For this review, use the dimensioned drawing (mm, ordinates from the lowest corner) and the shaded views. A direction names the side the tool comes from. Coordinates: 2 decimals unless noted, no trailing zeros. Order: outer loops, then holes, each group sorted by start corner. A loop starts at its lowest first (then second) coordinate and runs counter-clockwise, first axis right, second up. Notation, with made-up numbers: M 48,84 L 86,84 A27 ccw 86,106 Z; hole C 76,48.25 d9. An arc over 180 degrees is marked long. Answer in a Markdown table with one row per item.
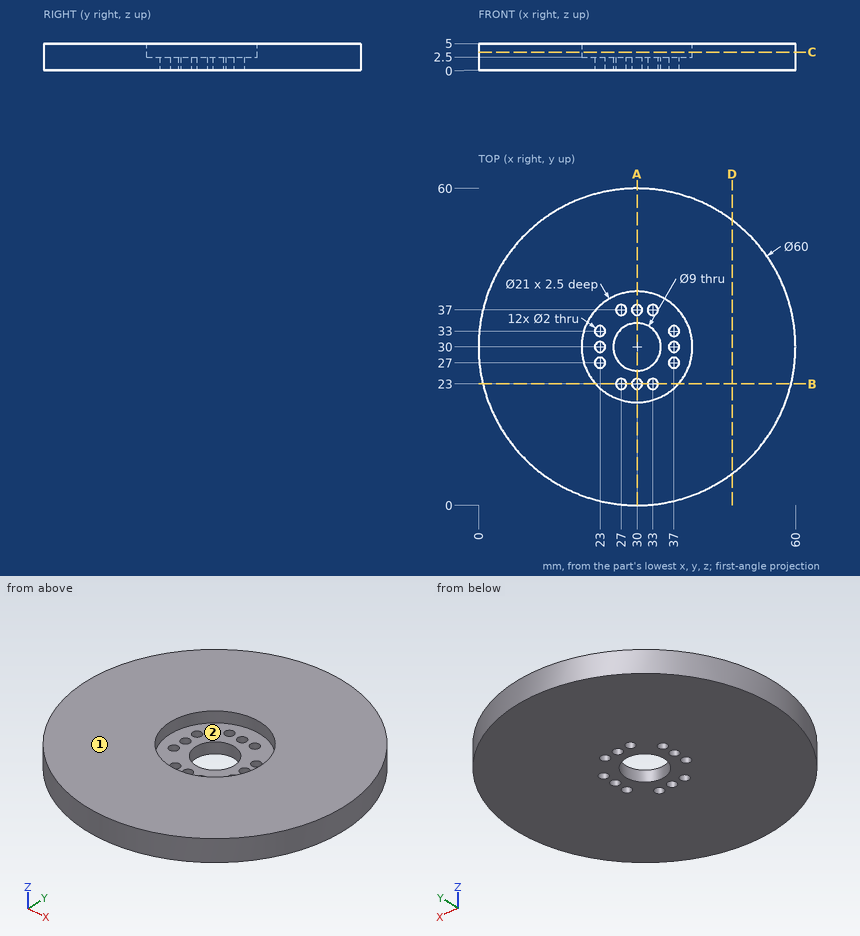
(1) Add section D-D, the plane x = 48. Give the boundary of the cut face in (y, z).
Return value:
| item | result |
|---|---|
| outline | M 6,0 L 54,0 L 54,5 L 6,5 Z |
(2) Insertion check: pin 1 Ø5.5 at (x, y) = (30, 30) entering from +Z; pin 2 Ø1.5 at (x, z) = (17.5, 1.5) entering from +Y; pin 3 Ø2.5 at (x, y) = (27, 37) entering from +Z; pin 4 Ø1 at (x, z) = (43, 2) entering from -Y. Each pin has a flat end and moves straight along its axis. Give the tip position at first contact, or say it passes through.
Return value:
| item | result |
|---|---|
| pin 1 | passes through |
| pin 2 | stops at y = 57.6 |
| pin 3 | stops at z = 2.5 |
| pin 4 | stops at y = 2.73 |
(3) For line 1 along Y through (x, z) = (30, 1.4); line 2 along Y through (x, z) = (29.5, 1.4); line 3 along Y through (x, z) = (30, 3.2), list the stretches that pass through material, from the lowest coordinate up. Write a range as from..to.
Return value:
| item | result |
|---|---|
| line 1 | y = 0..22, 24..25.5, 34.5..36, 38..60 |
| line 2 | y = 0..22.13, 23.87..25.53, 34.47..36.13, 37.87..60 |
| line 3 | y = 0..19.5, 40.5..60 |
(4) For the marked faces 1 and 2, list the 3-axis set-ups (+Z, -Z, +X, -X, +Y, -Y) from which the entire face can be reached by the end or side of a thin tool; tool diameter is ignored.
Return value:
| item | result |
|---|---|
| face 1 | +Z, +X, -X, +Y, -Y |
| face 2 | +Z |
(5) Add section A-A, the plane x = 30. Give the boundary of the cut face in (y, z).
Return value:
| item | result |
|---|---|
| outline | M 0,0 L 22,0 L 22,2.5 L 19.5,2.5 L 19.5,5 L 0,5 Z; M 24,0 L 25.5,0 L 25.5,2.5 L 24,2.5 Z; M 34.5,0 L 36,0 L 36,2.5 L 34.5,2.5 Z; M 38,0 L 60,0 L 60,5 L 40.5,5 L 40.5,2.5 L 38,2.5 Z |
(6) Add section C-C, the plane z = 3.45. Give the boundary of the cut face in (x, y), and give its area (3 significant figures).
Return value:
| item | result |
|---|---|
| outline | C 30,30 d60; hole C 30,30 d21 |
| area | 2,480 mm2 |
(7) Add section B-B, the plane y = 23. Give the boundary of the cut face in (x, z), and give its area (3 significant figures).
Return value:
| item | result |
|---|---|
| outline | M 0.83,0 L 26,0 L 26,2.5 L 22.17,2.5 L 22.17,5 L 0.83,5 Z; M 28,0 L 29,0 L 29,2.5 L 28,2.5 Z; M 31,0 L 32,0 L 32,2.5 L 31,2.5 Z; M 34,0 L 59.17,0 L 59.17,5 L 37.83,5 L 37.83,2.5 L 34,2.5 Z |
| area | 238 mm2 |
